```python
from build123d import *

# Parameters (mm, degrees)
REVOLUTION_ANGLE     = -54.075512
SKETCH002_W          = 49
SKETCH002_H          = 28
PAD_DEPTH            = 6
SKETCH003_W          = 35
SKETCH003_H          = 17
POCKET001_DEPTH      = 0.001
POCKET001_DEPTH_BACK = 33.411
SKETCH004_R          = 1.25
POCKET_DEPTH         = 3.1
SKETCH001_W          = 59
SKETCH001_H          = 38
SKETCH001_W_2        = 49
SKETCH001_H_2        = 28
POCKET005_DEPTH      = 5.778131
SKETCH009_R          = 11
POCKET006_DEPTH      = 33.411


with BuildPart() as part:
    # Sketch → Revolution (revolve, symmetric)
    with BuildSketch(Plane.XZ) as revolution_sk:
        Polygon((-3, 31.41), (46, 31.41), (46, 27.5), (18.2, 27.5), (18.2, 28.41), (0, 28.41), (0, 25.41), (-3, 25.41), align=None)
    revolve(axis=Axis((0, 0, 0), (1, 0, 0)), revolution_arc=REVOLUTION_ANGLE / 2)
    revolve(revolution_sk.sketch, axis=Axis((0, 0, 0), (-1, 0, 0)), revolution_arc=REVOLUTION_ANGLE / 2)

    # Sketch002 → Pad (new body)
    with BuildSketch(Plane.XY.offset(27.41)):
        with Locations((21.5, 0)):
            Rectangle(SKETCH002_W, SKETCH002_H)
    extrude(amount=PAD_DEPTH)

    # Sketch003 → Pocket001 (cut, two sides)
    with BuildSketch(Plane.XY) as pocket001_sk:
        with Locations((17.5, 0)):
            Rectangle(SKETCH003_W, SKETCH003_H)
    extrude(amount=-POCKET001_DEPTH, mode=Mode.SUBTRACT)
    extrude(pocket001_sk.sketch, amount=POCKET001_DEPTH_BACK, mode=Mode.SUBTRACT)

    # Sketch004 → Pocket (cut)
    with BuildSketch(Plane.XY.offset(33.51)):
        with Locations((43.75, 11.25)):
            Circle(SKETCH004_R)
        with Locations((0.25, 11.25)):
            Circle(SKETCH004_R)
        with Locations((0.25, -11.25)):
            Circle(SKETCH004_R)
        with Locations((43.75, -11.25)):
            Circle(SKETCH004_R)
    extrude(amount=-POCKET_DEPTH, mode=Mode.SUBTRACT)

    # Sketch001 → Pocket005 (cut, through all)
    with BuildSketch(Plane.XY.offset(28.41)):
        with Locations((21.5, 0)):
            Rectangle(SKETCH001_W, SKETCH001_H)
        with Locations((21.5, 0)):
            Rectangle(SKETCH001_W_2, SKETCH001_H_2, mode=Mode.SUBTRACT)
    extrude(amount=-POCKET005_DEPTH, mode=Mode.SUBTRACT)

    # Sketch009 → Pocket006 (cut, through all)
    with BuildSketch(Plane.XY):
        with Locations((22, 0)):
            Circle(SKETCH009_R)
    extrude(amount=POCKET006_DEPTH, mode=Mode.SUBTRACT)


solid = part.part
```
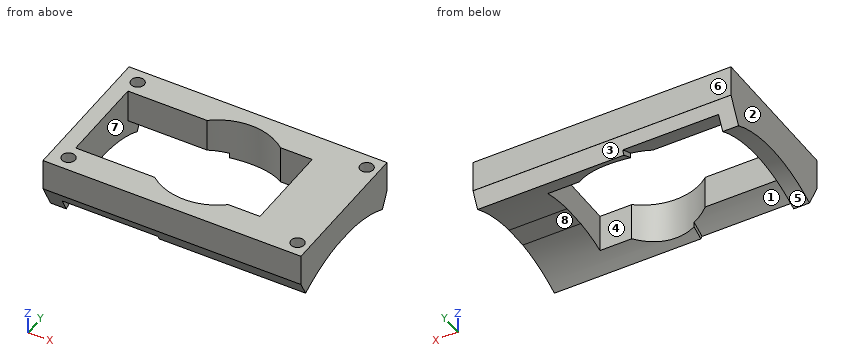
Verification items for the finished model (mm, model axes). Face numbers are marked on the shaded views. A direction names the side the tool comes from. Round coordinates to 2 decimals unless told otherwise and drop trailing zeros. Write each loop counter-clockwise with the first axis right and the second up, starting at its lowest first coordinate (ties: lowest second). Pieces come first, ordered by that corner, then holes. Notation, with made-up numbers: (-20.5, -24.75) -> (14.5, -24.75) arc R15 cw to (14.5, -20.75) -> close; hole circle Ø3 at (55.25, -24.75). An arc over 180 degrees is marked (long way). Write each question's results on one line, items separated by ' | '. Start each with the question number.
1. Set-up check for the marked faces 4, 5, 6, 7 and 8: record each of +Z, -Z, +X, -X, +Y, -Y from which the full face is reachable in a straight line by a thin tool's end or side.
2. Cross-section at C-C (y = 9). Enter the section's corners in (x, z), then the cut area to 3 significant figures.
3. Draft check along X on the marked faces 1, 2 and 3. Enter one of: +X half, -X half, draft (parallel to the pull), parting line (faces both ways), or undercut.
4. Cross-section at A-A (z = 32.75). Enter the section's corners in (x, y).
5. Material ranges on probe 1 along Y at (x, z) = (43.75, 32.8); probe 2 along Y at (x, z) = (0.25, 31.8); probe 3 along X at (y, z) = (-2.25, 29), recorded low to high. Write a range as from..to.
6. Depth check by flat-ended pin: P1, Ø1.2, axis at x = 0.5, y = -11, coming from the +Z side; P2, Ø2, axis at x = 40, y = 0, coming from the -Z side; P3, Ø3, axis at x = 43.75, y = -11.25, coming from the -Z side. Enter the tip coordinate at first touch or a pass-through.
Solutions:
1) face 4: +Z, -Z | face 5: -Z, +X, -X | face 6: +Z, -Z, +X, -X, +Y | face 7: -Z | face 8: -Z, +X
2) outline: (-3, 23.76) -> (0, 23.76) -> (0, 26.95) -> (15.68, 26.95) -> (15.68, 33.41) -> (-3, 33.41) -> close; (28.32, 25.99) -> (46, 25.99) -> (46, 33.41) -> (28.32, 33.41) -> close | area: 261 mm2
3) face 1: undercut | face 2: -X half | face 3: draft
4) outline: (-3, -14) -> (46, -14) -> (46, 14) -> (-3, 14) -> close; hole circle Ø2.5 at (0.25, -11.25); hole circle Ø2.5 at (0.25, 11.25); hole (0, -8.5) -> (15.02, -8.5) arc R11 ccw to (28.98, -8.5) -> (35, -8.5) -> (35, 8.5) -> (28.98, 8.5) arc R11 ccw to (15.02, 8.5) -> (0, 8.5) -> close; hole circle Ø2.5 at (43.75, -11.25); hole circle Ø2.5 at (43.75, 11.25)
5) probe 1: y = -14..-12.5, -10..10, 12.5..14 | probe 2: y = -14..-12.5, -10..-8.5, 8.5..10, 12.5..14 | probe 3: x = -3..0, 35..46
6) P1: stops at z = 30.41 | P2: stops at z = 27.41 | P3: stops at z = 24.49
